from build123d import *

# Parameters (mm, degrees)
F0_R     = 50.8
F1_DEPTH = 50.8
F2_R     = 48.26
F3_DEPTH = 45.72
F4_R     = 5.08
F5_R     = 5.08
F7_DEPTH = 50.8
F8_R     = 1.27


# Not quite as in the source:
# - the program builds the solid bodies; features that only make, move or delete a surface that nothing else refers to are left out


with BuildPart() as f1:
    # F0 (on Top) → F1 (new body)
    with BuildSketch(Plane.XY):
        Circle(F0_R)
    extrude(amount=F1_DEPTH)

    # F2 (on face) → F3 (cut)
    with BuildSketch(Plane.XY.offset(50.8)):
        Circle(F2_R)
    extrude(amount=-F3_DEPTH, mode=Mode.SUBTRACT)

    # F4
    f4_edges = [f1.edges().sort_by_distance(p)[0] for p in [
        (-48.26, 0, 5.08),
    ]]
    fillet(f4_edges, radius=F4_R)

    # F5
    f5_edges = [f1.edges().sort_by_distance(p)[0] for p in [
        (-50.8, 0, 0),
    ]]
    fillet(f5_edges, radius=F5_R)

    # F6 (on face) → F7 (join)
    with BuildSketch(Plane.XY.offset(50.8)):
        with BuildLine():
            ThreePointArc((5.08, 53.34), (0, 58.42), (-5.08, 53.34))
            Line((-5.08, 53.34), (-5.0849799889, 50.5448610495))
            ThreePointArc((-5.0849799889, 50.5448610495), (-0.002502551, 50.7999999384), (5.08, 50.545361805))
            Line((5.08, 50.545361805), (5.08, 50.8))
            Line((5.08, 50.8), (5.08, 53.34))
        make_face()
    extrude(amount=-F7_DEPTH)

    # F8
    f8_edges = [f1.edges().sort_by_distance(p)[0] for p in [
        (-0.002503, 50.8, 0),
    ]]
    fillet(f8_edges, radius=F8_R)


solid = f1.part
Read the model definition and answer for the solid it produces. Units are mm, in the model's axes. A direction names the side the tool comes from. Round coordinates to 2 decimals unless told otherwise and drop trailing zeros. Write each loop counter-clockwise with the first axis right and the second up, starting at its lowest first coordinate (ties: lowest second). Pieces come first, ordered by that corner, then holes. Notation, with made-up numbers: (66, 35.25) - (96, 35.25) arc R12 cw to (96, 58.25) - close; hole circle Ø1 at (78.25, -37). An arc over 180 degrees is marked (long way). Use a Markdown table: item, result.
(1) The part is cut by section A-A (z = 40). Write down the section's boundary in (x, y).
Reported:
| item | result |
|---|---|
| outline | (-5.08, 50.54) arc R50.8 ccw (long way) to (5.08, 50.55) - (5.08, 53.34) arc R5.08 ccw to (-5.08, 53.34) - close; hole circle Ø96.52 at (0, 0) |
(2) The mould has two halves that part along X. Classify faces 1 (the cylindrical face through (46.03, 14.5, 30.76)), 2 (the cylindrical face through (-2.16, -50.754, 27.62)), 3 (the flat face through (0, 54, 0)): released by +X, released by -X, zero draft, split by the parting line, or undercut.
Reported:
| item | result |
|---|---|
| face 1 | undercut |
| face 2 | split by the parting line |
| face 3 | zero draft |
(3) Which of the six approach directions +Z, -Z, +X, -X, +Y, -Y give full straight-line access (tool end or side, diameter ignored) to faces 4 (the cylindrical face through (0.11, 58.42, 25.76)), 5 (the flat face through (5.08, 52, 26)), 6 (the flat face through (-1, 1, 5.08))?
Reported:
| item | result |
|---|---|
| face 4 | +Z, -Z, +Y |
| face 5 | +Z, -Z, +X, +Y |
| face 6 | +Z |
(4) The part is cut by section B-B (y = 0). Write down the section's boundary in (x, z), then the cut area to 3 significant figures.
Reported:
| item | result |
|---|---|
| outline | (-50.8, 5.08) arc R5.08 ccw to (-45.72, 0) - (45.72, 0) arc R5.08 ccw to (50.8, 5.08) - (50.8, 50.8) - (48.26, 50.8) - (48.26, 10.16) arc R5.08 cw to (43.18, 5.08) - (-43.18, 5.08) arc R5.08 cw to (-48.26, 10.16) - (-48.26, 50.8) - (-50.8, 50.8) - close |
| area | 748 mm2 |
(5) Each of these flat-tipped pins is pushed along its axis until it touches: pin 1 Ø3 at (x, y) = (-30, 16) entering from +Z; pin 2 Ø12 at (y, z) = (-17, 32) entering from +X; pin 3 Ø0.8 at (y, z) = (52.5, 23) entering from +X. Where does it stop, or does it pass through?
Reported:
| item | result |
|---|---|
| pin 1 | z = 5.08 |
| pin 2 | x = 49.59 |
| pin 3 | x = 5.08 |
(6) Straight lines are drawn through the part: line 1 along Y through (x, z) = (0, 36); line 2 along Z through (x, y) = (-4, -22); line 3 along X through (y, z) = (-23, 22.5). For each, find the intervals that lie inside material, in ascending order. Write a range as [from, to].
Reported:
| item | result |
|---|---|
| line 1 | [-50.8, -48.26], [48.26, 58.42] |
| line 2 | [0, 5.08] |
| line 3 | [-45.3, -42.43], [42.43, 45.3] |
